Could you check a few things on this drawing? It's one solid part, dimensions in mm from its lowest x, y, z. Coordinates: 2 decimals unless noted, no trailing zeros. Order: outer loops, then holes, each group sorted by start corner. A loop starts at its lowest first (then second) coordinate and runs counter-clockwise, first axis right, second up. Notation, with made-up numbers: M -37,22.25 L 20,22.25 A13 cw 20,38.25 Z; hole C 16,27.5 d1. An arc over 180 degrees is marked long. Answer as CSV lines item,"result". Start each with the question number.
1. If we section it at C-C (z = 15.75): List the corners of the cut face in (x, y) for me.
2. If we section it at D-D (x = 34): List the corners of the cut face in (y, z) for me, plus the area to 3 significant figures.
3. I need wall thicknesses on line 1 along Y through (x, z) = (148.5, 3); line 2 along Y through (x, z) = (248, 1) (1 decimal); line 3 along X through (y, z) = (163, 4). Which ranges of each line are inside material? Lowest first, please. Write a range as from..to.
4. Will these pins go through, and if not, where does the flat tip stop? pin 1 (2 mm diameter, centred on y = 38, z = 4.5, fed in from -X); pin 2 (2 mm diameter, centred on y = 97.5, z = 15, fed in from -X); pin 3 (2 mm diameter, centred on y = 137, z = 6.5, fed in from +X).
5. If we section it at B-B (y = 208.5): List the corners of the cut face in (x, z) for me.
6. If we section it at A-A (x = 148.5): List the corners of the cut face in (y, z) for me.
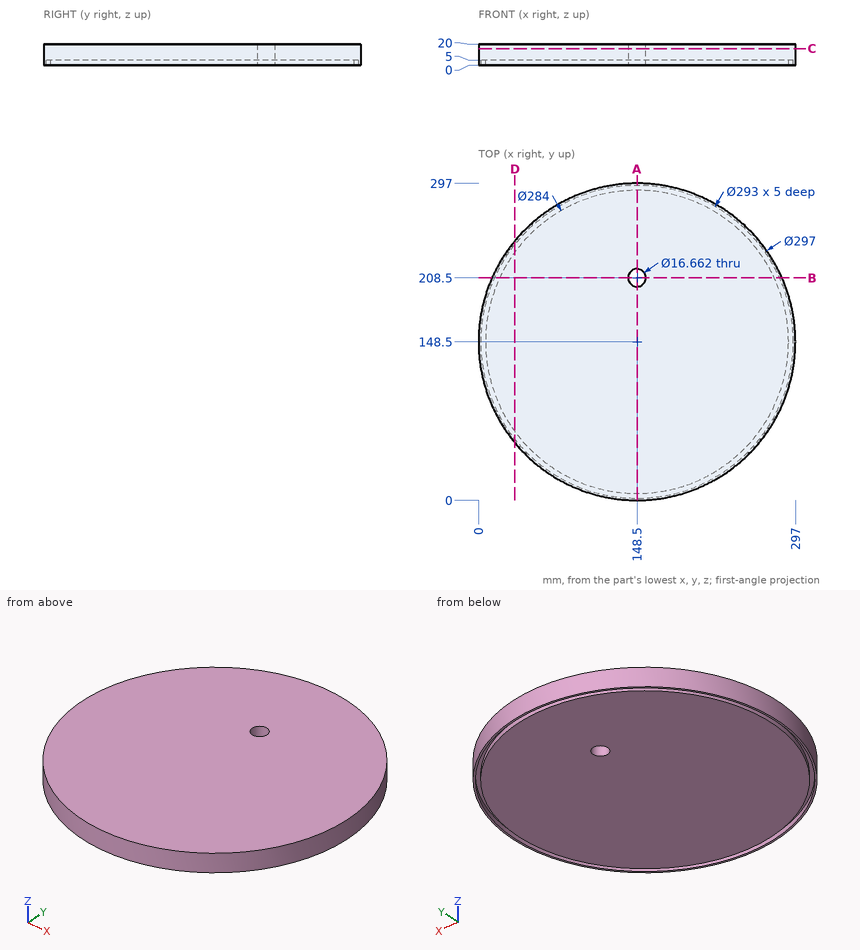
Solved:
1,outline,"C 148.5,148.5 d297; hole C 148.5,208.5 d16.66"
2,outline,"M 53.94,0 L 57.11,0 L 57.11,5 L 64.51,5 L 64.51,0 L 232.49,0 L 232.49,5 L 239.89,5 L 239.89,0 L 243.06,0 L 243.06,20 L 53.94,20 Z"
2,area,"3,710 mm²"
3,line 1,"0..2, 6.5..200.17, 216.83..290.5, 295..297"
3,line 2,"38.3..41, 47.2..249.8, 256..258.7"
3,line 3,"0.71..2.72, 7.24..289.76, 294.28..296.29"
4,pin 1,"x = 48.19"
4,pin 2,"x = 8.67"
4,pin 3,"x = 296.63"
5,outline,"M 12.66,0 L 14.85,0 L 14.85,5 L 19.8,5 L 19.8,0 L 140.17,0 L 140.17,20 L 12.66,20 Z; M 156.83,0 L 277.2,0 L 277.2,5 L 282.15,5 L 282.15,0 L 284.34,0 L 284.34,20 L 156.83,20 Z"
6,outline,"M 0,0 L 2,0 L 2,5 L 6.5,5 L 6.5,0 L 200.17,0 L 200.17,20 L 0,20 Z; M 216.83,0 L 290.5,0 L 290.5,5 L 295,5 L 295,0 L 297,0 L 297,20 L 216.83,20 Z"
